from build123d import *

# Parameters (mm, degrees)
F0_W     = 50
F0_H     = 50
F1_DEPTH = 20
F2_R     = 2
F3_R     = 18.791434
F4_DEPTH = 32.6
F6_R     = 19.635013
F7_DEPTH = 7.2


with BuildPart() as f1:
    # F0 (on Top) → F1 (new body)
    with BuildSketch(Plane.XY):
        with Locations((25, 25)):
            Rectangle(F0_W, F0_H)
    extrude(amount=F1_DEPTH)

    # F2
    f2_edges = [f1.edges().sort_by_distance(p)[0] for p in [
        (50, 25, 20),
        (25, 50, 20),
        (0, 25, 20),
        (25, 0, 20),
    ]]
    fillet(f2_edges, radius=F2_R)

    # F3 (on face) → F4 (join)
    with BuildSketch(Plane.XY.offset(20)):
        with Locations((25, 25)):
            Circle(F3_R)
    extrude(amount=-F4_DEPTH)

    # F6 (on face) → F7 (cut)
    with BuildSketch(Plane.XY.offset(20)):
        with Locations((25, 25.156734)):
            Circle(F6_R)
    extrude(amount=-F7_DEPTH, mode=Mode.SUBTRACT)


solid = f1.part
Geometry: final body of the model. Coordinates: model frame, mm. A direction names the side the tool comes from. Give positions to 0.01 mm unless a question says otherwise; leave off trailing zeros. Write each loop counter-clockwise with the first axis right and the second up, starting at its lowest first coordinate (ties: lowest second). Pieces come first, ordered by that corner, then holes.
(1) Mould query, pull axis Y, two halves, no side actions, for faces 1 (the flat face through (25, 25, 12.8)), 2 (the cylindrical face through (25.35, 49.43, 19.4)), 3 (the cylindrical face through (20.926, 6.655, -6.212)). Classes: released by +Y, released by -Y, zero draft, split by the parting line, or undercut.
(2) First-contact query: P1, Ø19.5, axis at x = 34, y = 28.5, coming from the +Z side; P2, Ø4, axis at x = 9, z = 14, coming from the -Y side. Flat tips, straight axial feed; report the tip coordinate or a pass-through.
(3) Ray query, line 1 (Y direction, x = 25, z = 16); line 2 (Z direction, x = 12, y = 9); line 3 (Z direction, x = 10.5, y = 21.5). Return the intervals inside material, ascending.
(4) Cut plane B-B, the plane z = -10. Return loops of the section in (x, y), then the cut area to 3 significant figures.
(5) Cut plane A-A, the plane x = 25. Return loops of the section in (y, z).
(6) Access query for faces 4 (the cylindrical face through (0.57, 25.35, 19.4)), 5 (the cylindrical face through (9.42, 13.21, 16.45)), 6 (the flat face through (36, 9, 0)). Directions: +Z, -Z, +X, -X, +Y, -Y. A direction counts if a zero-diameter tool reaches every point of the face in a straight line with its end or side. Return the directions, or none.
(7) Cut plane D-D, the plane z = 16. Return loops of the section in (x, y), then the cut area to 3 significant figures.
(8) Cut plane C-C, the plane y = 30. Return loops of the section in (x, z).
Values follow:
1. face 1: undercut
1. face 2: released by +Y
1. face 3: split by the parting line
2. P1: stops at z = 12.8
2. P2: stops at y = 0
3. line 1: y = 0 to 5.52, 44.79 to 50
3. line 2: z = 0 to 20
3. line 3: z = -12.6 to 12.8
4. outline: circle Ø37.58 at (25, 25)
4. area: 1,110 mm2
5. outline: (0, 0) - (6.21, 0) - (6.21, -12.6) - (43.79, -12.6) - (43.79, 0) - (50, 0) - (50, 18) arc R2 ccw to (48, 20) - (44.79, 20) - (44.79, 12.8) - (5.52, 12.8) - (5.52, 20) - (2, 20) arc R2 ccw to (0, 18) - close
6. face 4: +Z, -X, +Y, -Y
6. face 5: +Z
6. face 6: -Z
7. outline: (0, 0) - (50, 0) - (50, 50) - (0, 50) - close; hole circle Ø39.27 at (25, 25.16)
7. area: 1,290 mm2
8. outline: (0, 0) - (6.89, 0) - (6.89, -12.6) - (43.11, -12.6) - (43.11, 0) - (50, 0) - (50, 18) arc R2 ccw to (48, 20) - (44.03, 20) - (44.03, 12.8) - (5.97, 12.8) - (5.97, 20) - (2, 20) arc R2 ccw to (0, 18) - close
